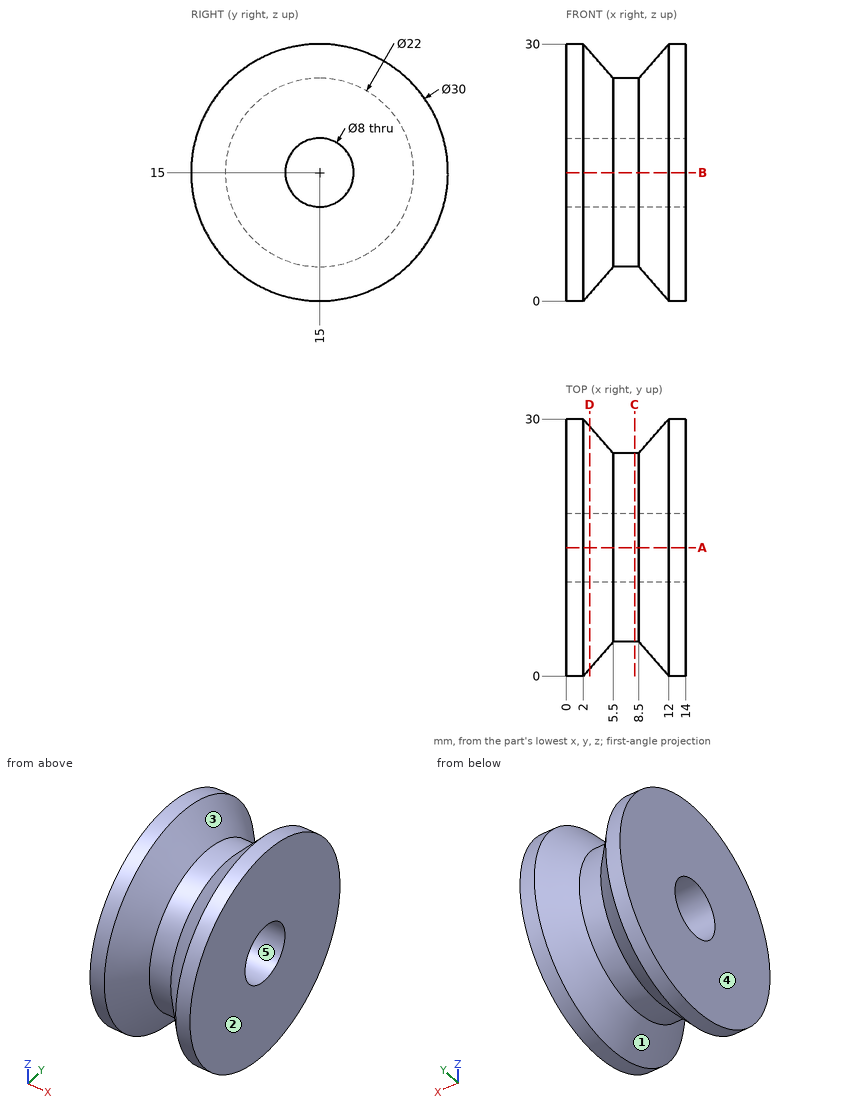
The figure shows three views and two pictorial views of one solid part (mm, origin at its lowest corner). Answer the questions. A direction names the side the tool comes from. Coordinates: 2 decimals unless noted, no trailing zeros. Order: outer loops, then holes, each group sorted by start corner. A loop starts at its lowest first (then second) coordinate and runs counter-clockwise, first axis right, second up.
Q1. Given P1, Ø5, axis at x = 3.5, z = 16.5, coming from the +Y side; P2, Ø2, axis at x = 9.5, z = 26, coming from the -Y side; P3, Ø4, axis at x = 3.5, z = 19.5, coming from the -Y side; P4, Ø6, axis at x = 8, z = 11.5, coming from the -Y side, each flat-ended and moving along its own axis, determine where each tip first touches the part or whether it passes through.
Q2. A cutting plane is placed at C-C, the plane x = 8. Write down the section's boundary in (y, z).
Q3. For a pull along Y with two mould halves and no side action, classify the marked faces 3, 4 and 5 as pulls with the +Y half, pulls with the -Y half, needs draft (parallel to the pull), parting line crosses it, or undercut.
Q4. A cutting plane is placed at A-A, the plane y = 15. Write down the section's boundary in (x, z), and give its area (3 significant figures).
Q5. A cutting plane is placed at D-D, the plane x = 2.75. Write down the section's boundary in (y, z), and give its area (3 significant figures).
Q6. Consider line 1 (Z direction, x = 5.75, y = 15); line 2 (Y direction, x = 12, z = 14.75); line 3 (Y direction, x = 5.25, z = 15.5). Determine where each line is inside the solid, lowest interval first.
Q7. Which of the six approach directions +Z, -Z, +X, -X, +Y, -Y give full straight-line access (tool end or side, diameter ignored) to the marked faces 1 and 2?
Answers follow:
1. P1: stops at y = 30
1. P2: stops at y = 7.1
1. P3: stops at y = 0.34
1. P4: stops at y = 1.52
2. outline: circle Ø22 at (15, 15); hole circle Ø8 at (15, 15)
3. face 3: parting line crosses it
3. face 4: needs draft
3. face 5: undercut
4. outline: (0, 0) - (2, 0) - (5.5, 4) - (8.5, 4) - (12, 0) - (14, 0) - (14, 11) - (0, 11) - close; (0, 19) - (14, 19) - (14, 30) - (12, 30) - (8.5, 26) - (5.5, 26) - (2, 30) - (0, 30) - close
4. area: 256 mm2
5. outline: circle Ø28.29 at (15, 15); hole circle Ø8 at (15, 15)
5. area: 578 mm2
6. line 1: z = 4 to 11, 19 to 26
6. line 2: y = 0 to 11.01, 18.99 to 30
6. line 3: y = 3.73 to 11.03, 18.97 to 26.27
7. face 1: none
7. face 2: +Z, -Z, +X, +Y, -Y
